```python
from build123d import *

# Parameters (mm, degrees)
F0_R     = 292.1
F1_DEPTH = 53.975
F2_R     = 206.375
F3_DEPTH = 1.5875
F4_R     = 212.725
F5_DEPTH = 22.225
F5_TAPER = 3
F6_R     = 180
F7_DEPTH = 77.7885001
F9_D     = 31.75


with BuildPart() as f1:
    # F0 (on Top) → F1 (new body)
    with BuildSketch(Plane.XY):
        Circle(F0_R)
    extrude(amount=-F1_DEPTH)

    # F2 (on face) → F3 (join)
    with BuildSketch(Plane.XY):
        Circle(F2_R)
    extrude(amount=F3_DEPTH)

    # F4 (on face) → F5 (join)
    with BuildSketch(Plane(origin=(0, 0, -53.975), x_dir=(1, 0, 0), z_dir=(0, 0, -1))):
        Circle(F4_R)
    extrude(amount=F5_DEPTH, taper=F5_TAPER)

    # F6 (on face) → F7 (cut, through all)
    with BuildSketch(Plane.XY.offset(1.5875)):
        with Locations((6.9869458067, 0)):
            Circle(F6_R)
    extrude(amount=-F7_DEPTH, mode=Mode.SUBTRACT)

    # F9 (through all)
    with Locations(Plane.XY):
        with Locations((244.5879595782, 79.4714455284), (208.0589455284, 151.1636722583), (151.1636722583, 208.0589455284), (79.4714455284, 244.5879595782), (0, 257.175), (-79.4714455284, 244.5879595782), (-151.1636722583, 208.0589455284), (-208.0589455284, 151.1636722583), (-244.5879595782, 79.4714455284), (-257.175, 0), (-244.5879595782, -79.4714455284), (-208.0589455284, -151.1636722583), (-151.1636722583, -208.0589455284), (-79.4714455284, -244.5879595782), (0, -257.175), (79.4714455284, -244.5879595782), (151.1636722583, -208.0589455284), (208.0589455284, -151.1636722583), (244.5879595782, -79.4714455284), (257.175, 0)):
            Hole(F9_D / 2)


solid = f1.part
```
For this review, take the finished solid that the model builds, in its own axes (mm). A direction names the side the tool comes from. Give positions to 0.01 mm unless a question says otherwise; leave off trailing zeros.
Item 1: Insertion check: P1, Ø6, axis at y = 136, z = -61.5, coming from the -X side; P2, Ø3, axis at x = -37, z = -43.5, coming from the +Y side; P3, Ø4, axis at x = -129, z = -58, coming from the -Y side. Each pin has a flat end and moves straight along its axis. Give the tip position at first contact, or say it passes through.
Item 2: Machinability: for faces 4 (the face through (-163.77, -125.58, 0.78)), 5 (the face through (278.61, 87.74, -26.61)), which of the approach directions +Z, -Z, +X, -X, +Y, -Y give a long, thin tool a straight path to every point of the face, cutting with its end or side? Answer none if there is none.
Item 3: The part is to be moulded in two halves that separate along X. For faces 1 (the face through (-169, 47, 1.588)), 2 (the face through (-27.548, -209.816, -75.121)), 3 (the face through (154.605, 192.561, -27.365)), say which applies: +X half, -X half, draft (parallel to the pull), parting line (faces both ways), or undercut.
Item 4: Take a section at A-A (x = 0). Give the number of separate pieces and of enclosed holes in the cut face, and give its area (3 significant figures).
Item 5: Wall thickness on probe 1 along X at (y, z) = (-221.5, -51.5); probe 2 along Y at (x, z) = (-83, -4.5); probe 3 along Y at (x, z) = (257.5, -13): over which ranges is each line inside the solid? List them lowest first.
Established:
1. P1: stops at x = -165.52
1. P2: stops at y = 289.93
1. P3: stops at y = -170.4
2. face 4: +Z
2. face 5: +Z, -Z
3. face 1: draft
3. face 2: parting line
3. face 3: undercut
4. separate pieces: 4
4. enclosed holes: 0
4. area: 10,200 mm2
5. probe 1: x = -190.42 to -159.61, -142.72 to 142.72, 159.61 to 190.42
5. probe 2: y = -280.06 to -260.07, -229.11 to -155.89, 155.89 to 229.11, 260.07 to 280.06
5. probe 3: y = -137.9 to -88.71, -70.24 to -15.87, 15.87 to 70.24, 88.71 to 137.9
